The listing builds one solid part. Answer for the finished solid, in the listing's coordinates (mm). Face numbers are marked on the shaded views. A direction names the side the tool comes from. Coordinates: 2 decimals unless noted, no trailing zeros. Write each loop counter-clockwise with the first axis right and the second up, starting at its lowest first coordinate (ties: lowest second). Pieces come first, ordered by that corner, then holes. Notation, with made-up numbers: M 84,1.25 L 115,1.25 A30 cw 115,26.25 Z; hole C -13,-39.75 d5. An arc over 180 degrees is marked long. Answer as CSV lines item,"result". Start each with the question number.
```python
from build123d import *
from build123d.topology import SkipClean

# Parameters (mm, degrees)
SKETCH_1_W          = 40
SKETCH_1_H          = 40
SKETCH_1_R          = 6.25
EXTRUDE_1_DEPTH     = 1.85
SKETCH_2_W          = 40
SKETCH_2_H          = 1
EXTRUDE_2_DEPTH     = 9.15
SKETCH_3_R          = 1.75
SKETCH_3_R_2        = 6.25
CUT_EXTRUDE_5_DEPTH = 31.347981811
SKETCH_4_R          = 7.255719344
CUT_EXTRUDE_6_DEPTH = 16.15


with BuildPart() as part:
    # 草图1 → 凸台-拉伸1 (new body)
    with BuildSketch(Plane.XY):
        Rectangle(SKETCH_1_W, SKETCH_1_H)
        Circle(SKETCH_1_R, mode=Mode.SUBTRACT)
    extrude(amount=EXTRUDE_1_DEPTH)

    # 草图2 → 凸台-拉伸2 (add)
    with BuildSketch(Plane.XY.offset(1.85)):
        with Locations((0, 19.5)):
            Rectangle(SKETCH_2_W, SKETCH_2_H)
        with Locations((0, 16.5)):
            Rectangle(SKETCH_2_W, SKETCH_2_H)
        with Locations((0, 13.5)):
            Rectangle(SKETCH_2_W, SKETCH_2_H)
        with Locations((0, 10.5)):
            Rectangle(SKETCH_2_W, SKETCH_2_H)
        with Locations((0, 7.5)):
            Rectangle(SKETCH_2_W, SKETCH_2_H)
        with Locations((0, 4.5)):
            Rectangle(SKETCH_2_W, SKETCH_2_H)
        with Locations((0, 1.5)):
            Rectangle(SKETCH_2_W, SKETCH_2_H)
        with Locations((0, -1.5)):
            Rectangle(SKETCH_2_W, SKETCH_2_H)
        with Locations((0, -4.5)):
            Rectangle(SKETCH_2_W, SKETCH_2_H)
        with Locations((0, -7.5)):
            Rectangle(SKETCH_2_W, SKETCH_2_H)
        with Locations((0, -10.5)):
            Rectangle(SKETCH_2_W, SKETCH_2_H)
        with Locations((0, -13.5)):
            Rectangle(SKETCH_2_W, SKETCH_2_H)
        with Locations((0, -16.5)):
            Rectangle(SKETCH_2_W, SKETCH_2_H)
        with Locations((0, -19.5)):
            Rectangle(SKETCH_2_W, SKETCH_2_H)
    extrude(amount=EXTRUDE_2_DEPTH)

    # 草图3 → 切除-拉伸5 (cut, through all)
    with SkipClean():  # the faces are left unmerged after this step: merging them gives an invalid solid
        with BuildSketch(Plane(origin=(0, 0, 0), x_dir=(-1, 0, 0), z_dir=(0, 0, -1))):
            with Locations((-15.5, -15.5)):
                Circle(SKETCH_3_R)
            with Locations((15.5, -15.5)):
                Circle(SKETCH_3_R)
            with Locations(Location((0, 0, 0), (0, 0, 350.793103779))):
                Circle(SKETCH_3_R_2)
        extrude(amount=-CUT_EXTRUDE_5_DEPTH, mode=Mode.SUBTRACT)

    # 草图4 → 切除-拉伸6 (cut)
    with SkipClean():  # the faces are left unmerged after this step: merging them gives an invalid solid
        with BuildSketch(Plane.XY.offset(1.85)):
            with Locations((-15.5, -15.5)):
                Circle(SKETCH_4_R)
            with Locations((15.5, -15.5)):
                Circle(SKETCH_4_R)
        extrude(amount=CUT_EXTRUDE_6_DEPTH, mode=Mode.SUBTRACT)


solid = part.part
```
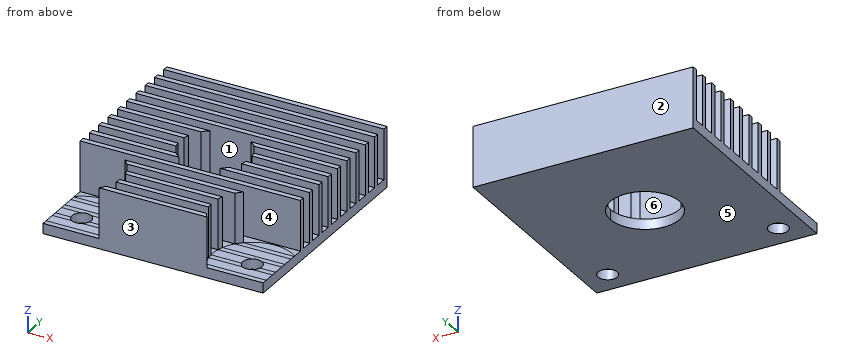
1) Which of the six approach directions +Z, -Z, +X, -X, +Y, -Y give full straight-line access (tool end or side, diameter ignored) to the marked faces 1 and 2?
2) The part is cut by section C-C (z = 10.5). Count the separate pieces of the cut face and the enclosed holes in it, then the cut area to 3 significant figures.
3) The part is cut by section B-B (z = 1.25). Determine the outline of the cut face in (x, y).
4) Find the intervals of material crossed by line 1 (X direction, y = -15.5, z = 1.1); line 2 (X direction, y = 0, z = 0.7); line 3 (Y direction, x = -15.5, z = 0.8), in increasing order. Write a range as from..to.
5) For a pull along Y with two mould halves and no side action, classify the marked faces 3, 4, 5 and 6 as +Y half, -Y half, draft (parallel to the pull), parting line (faces both ways), or undercut.
6) Each of these flat-tipped pins is pushed along its axis until it touches: P1, Ø5, axis at y = -3, z = 4.5, coming from the -X side; P2, Ø1, axis at x = -10.5, y = 0, coming from the +Z side. Where does it stop, or does it pass through?
7) The part is cut by section D-D (y = -3). Determine the outline of the cut face in (x, z), then the cut area to 3 significant figures.
8) The part is cut by section A-A (y = -15.5). Determine the outline of the cut face in (x, z).
Completed:
1,face 1,"+Z, +X, -X"
1,face 2,"+Z, -Z, +X, -X, +Y"
2,separate pieces,"18"
2,enclosed holes,"0"
2,area,"432 mm²"
3,outline,"M -20,-20 L 20,-20 L 20,20 L -20,20 Z; hole C -15.5,-15.5 d3.5; hole C 0,0 d12.5; hole C 15.5,-15.5 d3.5"
4,line 1,"-20..-17.25, -13.75..13.75, 17.25..20"
4,line 2,"-20..-6.25, 6.25..20"
4,line 3,"-20..-17.25, -13.75..20"
5,face 3,"-Y half"
5,face 4,"undercut"
5,face 5,"draft"
5,face 6,"undercut"
6,P1,"x = -20"
6,P2,"z = 1.85"
7,outline,"M -20,0 L -5.48,0 L -5.48,1.85 L -20,1.85 Z; M 5.48,0 L 20,0 L 20,1.85 L 5.48,1.85 Z"
7,area,"53.7 mm²"
8,outline,"M -20,0 L -17.25,0 L -17.25,1.85 L -20,1.85 Z; M -13.75,0 L 13.75,0 L 13.75,1.85 L -13.75,1.85 Z; M 17.25,0 L 20,0 L 20,1.85 L 17.25,1.85 Z"
